Geometry: final body of the model. Coordinates: model frame, mm. Face numbers are marked on the shaded views. A direction names the side the tool comes from. Give positions to 0.01 mm unless a question says otherwise; leave off trailing zeros. Loops run counter-clockwise (first coordinate to the right, second up) from the corner with the lowest first, then second, coordinate; pieces in that order, holes last.
1. Section B-B, the plane z = 10.5. Output: boundary loops of the cut face in (x, y).
2. First-contact query: P1, Ø4, axis at x = -30.5, y = 10.5, coming from the -Z side; P2, Ø2, axis at x = -40.5, y = 1.5, coming from the -Z side; P3, Ø11.5, axis at y = 9.65, z = 15.68, coming from the +X side; P4, Ø2, axis at x = -32.5, y = 16.5, coming from the -Z side. Flat tips, straight axial feed; report the tip coordinate or a pass-through.
3. Material intervals for line 1 along Z through (x, y) = (-38, 0.5); line 2 along Z through (x, y) = (-38, 18.75); line 3 along Y through (x, z) = (-41, 26.5), sorted ascending.
4. Section A-A, the plane y = 11.75. Output: boundary loops of the cut face in (x, z).
5. Draft query along Y for the marked faces 1, 2 and 3. Return one class per face: +Y half, -Y half, draft (parallel to the pull), parting line (faces both ways), or undercut.
6. Access query for the marked faces 4, 5 and 6. Directions: +Z, -Z, +X, -X, +Y, -Y. A direction counts if a zero-diameter tool reaches every point of the face in a straight line with its end or side. Return the directions, or none.
7. Section C-C, the plane y = -2. Output: boundary loops of the cut face in (x, z), then the cut area to 3 significant figures.
8. Section D-D, the plane z = 15.5. Output: boundary loops of the cut face in (x, y), then the cut area to 3 significant figures.
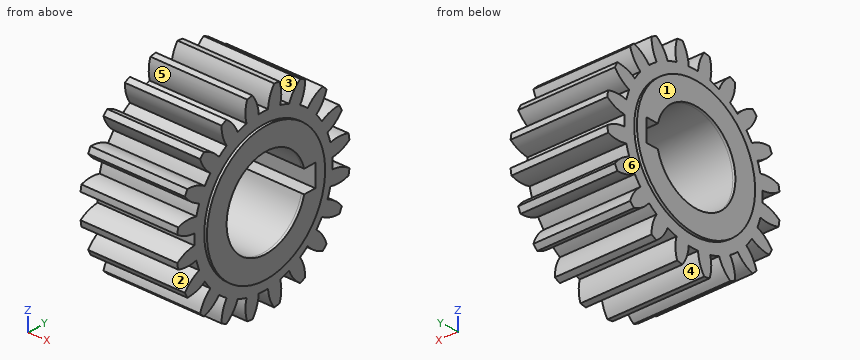
from build123d import *

# Parameters (mm, degrees)
SPUR_START             = -42.145535126
SPUR_GEAR_AI_OUTLINE_R = 6.35
SPUR_GEAR_AI_DEPTH     = 13.97
SKETCH1_W              = 3.175
SKETCH1_H              = 3.175
CUT_EXTRUDE1_DEPTH     = 41.258239372
SKETCH2_R              = 9.525
BOSS_EXTRUDE1_DEPTH    = 0.381
BOSS_EXTRUDE2_START    = 0.381
SKETCH3_R              = 9.525
BOSS_EXTRUDE2_DEPTH    = 0.381


# Read off the part's stored shape, not the designer's step: spur gear_ai
with BuildPart() as part:
    # spur gear_ai outline → spur gear_ai (new body)
    with BuildSketch(Plane.YZ.offset(SPUR_START)):
        with BuildLine():
            ThreePointArc((21.89573329, 8.949900066), (22.10150024, 9.338497576), (22.294935451, 9.733378421))
            ThreePointArc((22.294935451, 9.733378421), (21.269289936, 10.804918767), (19.977842952, 11.534516))
            ThreePointArc((19.977842952, 11.534516), (20.234833052, 12.242868992), (20.443283136, 12.966993591))
            ThreePointArc((20.443283136, 12.966993591), (21.916932187, 12.79815666), (23.376532451, 13.062191702))
            ThreePointArc((23.376532451, 13.062191702), (23.452145215, 13.495355381), (23.514088141, 13.93068415))
            ThreePointArc((23.514088141, 13.93068415), (22.207517114, 14.632837684), (20.7538201, 14.927646821))
            ThreePointArc((20.7538201, 14.927646821), (20.779339097, 15.680744858), (20.7538201, 16.433842895))
            ThreePointArc((20.7538201, 16.433842895), (22.207517114, 16.728652032), (23.514088141, 17.430805566))
            ThreePointArc((23.514088141, 17.430805566), (23.452145215, 17.866134334), (23.376532451, 18.299298013))
            ThreePointArc((23.376532451, 18.299298013), (21.916932187, 18.563333056), (20.443283136, 18.394496125))
            ThreePointArc((20.443283136, 18.394496125), (20.234833052, 19.118620724), (19.977842952, 19.826973715))
            ThreePointArc((19.977842952, 19.826973715), (21.269289936, 20.556570948), (22.294935451, 21.628111294))
            ThreePointArc((22.294935451, 21.628111294), (22.10150024, 22.022992139), (21.89573329, 22.41158965))
            ThreePointArc((21.89573329, 22.41158965), (20.425979632, 22.21166061), (19.07662958, 21.595704547))
            ThreePointArc((19.07662958, 21.595704547), (18.654614962, 22.219973346), (18.191309741, 22.814242767))
            ThreePointArc((18.191309741, 22.814242767), (19.194090867, 23.907210035), (19.83841354, 25.243247358))
            ThreePointArc((19.83841354, 25.243247358), (19.53242083, 25.559026591), (19.216641597, 25.865019301))
            ThreePointArc((19.216641597, 25.865019301), (17.880604274, 25.220696628), (16.787637006, 24.217915502))
            ThreePointArc((16.787637006, 24.217915502), (16.193367585, 24.681220723), (15.569098786, 25.103235341))
            ThreePointArc((15.569098786, 25.103235341), (16.185054849, 26.452585393), (16.384983889, 27.922339051))
            ThreePointArc((16.384983889, 27.922339051), (15.996386378, 28.128106001), (15.601505533, 28.321541212))
            ThreePointArc((15.601505533, 28.321541212), (14.529965187, 27.295895697), (13.800367954, 26.004448713))
            ThreePointArc((13.800367954, 26.004448713), (13.092014963, 26.261438813), (12.367890364, 26.469888897))
            ThreePointArc((12.367890364, 26.469888897), (12.536727295, 27.943537948), (12.272692252, 29.403138212))
            ThreePointArc((12.272692252, 29.403138212), (11.839528573, 29.478750976), (11.404199805, 29.540693902))
            ThreePointArc((11.404199805, 29.540693902), (10.702046271, 28.234122875), (10.407237134, 26.780425861))
            ThreePointArc((10.407237134, 26.780425861), (9.654139097, 26.805944858), (8.90104106, 26.780425861))
            ThreePointArc((8.90104106, 26.780425861), (8.606231923, 28.234122875), (7.904078389, 29.540693902))
            ThreePointArc((7.904078389, 29.540693902), (7.46874962, 29.478750976), (7.035585941, 29.403138212))
            ThreePointArc((7.035585941, 29.403138212), (6.771550899, 27.943537948), (6.94038783, 26.469888897))
            ThreePointArc((6.94038783, 26.469888897), (6.216263231, 26.261438813), (5.507910239, 26.004448713))
            ThreePointArc((5.507910239, 26.004448713), (4.778313006, 27.295895697), (3.70677266, 28.321541212))
            ThreePointArc((3.70677266, 28.321541212), (3.311891815, 28.128106001), (2.923294305, 27.922339051))
            ThreePointArc((2.923294305, 27.922339051), (3.123223344, 26.452585393), (3.739179408, 25.103235341))
            ThreePointArc((3.739179408, 25.103235341), (3.114910608, 24.681220723), (2.520641187, 24.217915502))
            ThreePointArc((2.520641187, 24.217915502), (1.427673919, 25.220696628), (0.091636597, 25.865019301))
            ThreePointArc((0.091636597, 25.865019301), (-0.224142637, 25.559026591), (-0.530135347, 25.243247358))
            ThreePointArc((-0.530135347, 25.243247358), (0.114187326, 23.907210035), (1.116968452, 22.814242767))
            ThreePointArc((1.116968452, 22.814242767), (0.653663231, 22.219973346), (0.231648613, 21.595704547))
            ThreePointArc((0.231648613, 21.595704547), (-1.117701439, 22.21166061), (-2.587455096, 22.41158965))
            ThreePointArc((-2.587455096, 22.41158965), (-2.793222046, 22.022992139), (-2.986657258, 21.628111294))
            ThreePointArc((-2.986657258, 21.628111294), (-1.961011743, 20.556570948), (-0.669564759, 19.826973715))
            ThreePointArc((-0.669564759, 19.826973715), (-0.926554858, 19.118620723), (-1.135004943, 18.394496125))
            ThreePointArc((-1.135004943, 18.394496125), (-2.608653994, 18.563333056), (-4.068254258, 18.299298013))
            ThreePointArc((-4.068254258, 18.299298013), (-4.143867021, 17.866134334), (-4.205809948, 17.430805566))
            ThreePointArc((-4.205809948, 17.430805566), (-2.899238921, 16.728652032), (-1.445541907, 16.433842895))
            ThreePointArc((-1.445541907, 16.433842895), (-1.471060903, 15.680744858), (-1.445541907, 14.927646821))
            ThreePointArc((-1.445541907, 14.927646821), (-2.899238921, 14.632837684), (-4.205809948, 13.93068415))
            ThreePointArc((-4.205809948, 13.93068415), (-4.143867021, 13.495355381), (-4.068254258, 13.062191702))
            ThreePointArc((-4.068254258, 13.062191702), (-2.608653994, 12.79815666), (-1.135004943, 12.966993591))
            ThreePointArc((-1.135004943, 12.966993591), (-0.926554858, 12.242868992), (-0.669564759, 11.534516))
            ThreePointArc((-0.669564759, 11.534516), (-1.961011743, 10.804918767), (-2.986657258, 9.733378421))
            ThreePointArc((-2.986657258, 9.733378421), (-2.793222046, 9.338497576), (-2.587455096, 8.949900066))
            ThreePointArc((-2.587455096, 8.949900066), (-1.117701439, 9.149829105), (0.231648613, 9.765785169))
            ThreePointArc((0.231648613, 9.765785169), (0.653663231, 9.141516369), (1.116968452, 8.547246948))
            ThreePointArc((1.116968452, 8.547246948), (0.114187326, 7.45427968), (-0.530135347, 6.118242358))
            ThreePointArc((-0.530135347, 6.118242358), (-0.224142637, 5.802463124), (0.091636597, 5.496470414))
            ThreePointArc((0.091636597, 5.496470414), (1.427673919, 6.140793087), (2.520641187, 7.143574213))
            ThreePointArc((2.520641187, 7.143574213), (3.114910608, 6.680268992), (3.739179408, 6.258254374))
            ThreePointArc((3.739179408, 6.258254374), (3.123223344, 4.908904322), (2.923294305, 3.439150665))
            ThreePointArc((2.923294305, 3.439150665), (3.311891815, 3.233383715), (3.70677266, 3.039948503))
            ThreePointArc((3.70677266, 3.039948503), (4.778313006, 4.065594018), (5.507910239, 5.357041002))
            ThreePointArc((5.507910239, 5.357041002), (6.216263231, 5.100050903), (6.94038783, 4.891600818))
            ThreePointArc((6.94038783, 4.891600818), (6.771550899, 3.417951767), (7.035585941, 1.958351503))
            ThreePointArc((7.035585941, 1.958351503), (7.46874962, 1.882738739), (7.904078389, 1.820795813))
            ThreePointArc((7.904078389, 1.820795813), (8.606231923, 3.12736684), (8.90104106, 4.581063854))
            ThreePointArc((8.90104106, 4.581063854), (9.654139097, 4.555544858), (10.407237134, 4.581063854))
            ThreePointArc((10.407237134, 4.581063854), (10.702046271, 3.12736684), (11.404199805, 1.820795813))
            ThreePointArc((11.404199805, 1.820795813), (11.839528573, 1.882738739), (12.272692252, 1.958351503))
            ThreePointArc((12.272692252, 1.958351503), (12.536727295, 3.417951767), (12.367890364, 4.891600818))
            ThreePointArc((12.367890364, 4.891600818), (13.092014962, 5.100050903), (13.800367954, 5.357041002))
            ThreePointArc((13.800367954, 5.357041002), (14.529965187, 4.065594018), (15.601505533, 3.039948503))
            ThreePointArc((15.601505533, 3.039948503), (15.996386378, 3.233383715), (16.384983889, 3.439150665))
            ThreePointArc((16.384983889, 3.439150665), (16.185054849, 4.908904322), (15.569098786, 6.258254374))
            ThreePointArc((15.569098786, 6.258254374), (16.193367585, 6.680268992), (16.787637006, 7.143574213))
            ThreePointArc((16.787637006, 7.143574213), (17.880604274, 6.140793087), (19.216641597, 5.496470414))
            ThreePointArc((19.216641597, 5.496470414), (19.53242083, 5.802463124), (19.83841354, 6.118242358))
            ThreePointArc((19.83841354, 6.118242358), (19.194090867, 7.45427968), (18.191309741, 8.547246948))
            ThreePointArc((18.191309741, 8.547246948), (18.654614962, 9.141516369), (19.07662958, 9.765785169))
            ThreePointArc((19.07662958, 9.765785169), (20.425979632, 9.149829105), (21.89573329, 8.949900066))
        make_face()
        with Locations((9.654139097, 15.680744858)):
            Circle(SPUR_GEAR_AI_OUTLINE_R, mode=Mode.SUBTRACT)
    extrude(amount=SPUR_GEAR_AI_DEPTH)

    # Sketch1 → Cut-Extrude1 (cut, through all)
    with BuildSketch(Plane(origin=(-28.175535126, 0, 0), x_dir=(0, 0, -1), z_dir=(1, 0, 0))):
        with Locations((-15.680744858, 16.004139097)):
            Rectangle(SKETCH1_W, SKETCH1_H)
    extrude(amount=-CUT_EXTRUDE1_DEPTH, mode=Mode.SUBTRACT)

    # Sketch2 → Boss-Extrude1 (add)
    with BuildSketch(Plane(origin=(-28.175535126, 0, 0), x_dir=(0, 0, -1), z_dir=(1, 0, 0))):
        with Locations(Location((-15.680744858, 9.654139097, 0), (0, 0, 180))):
            Circle(SKETCH2_R)
        with BuildLine():
            Line((-14.093244858, 17.591639097), (-17.268244858, 17.591639097))
            Line((-17.268244858, 17.591639097), (-17.268244858, 15.802500159))
            ThreePointArc((-17.268244858, 15.802500159), (-15.680744858, 3.304139097), (-14.093244858, 15.802500159))
            Line((-14.093244858, 15.802500159), (-14.093244858, 17.591639097))
        make_face(mode=Mode.SUBTRACT)
    extrude(amount=BOSS_EXTRUDE1_DEPTH)

    # Sketch3 → Boss-Extrude2 (add)
    with BuildSketch(Plane.ZY.offset(42.145535126).offset(BOSS_EXTRUDE2_START)):
        with Locations((15.680744858, 9.654139097)):
            Circle(SKETCH3_R)
        with BuildLine():
            Line((14.093244858, 15.802500159), (14.093244858, 17.591639097))
            Line((14.093244858, 17.591639097), (17.268244858, 17.591639097))
            Line((17.268244858, 17.591639097), (17.268244858, 15.802500159))
            ThreePointArc((17.268244858, 15.802500159), (15.680744858, 3.304139097), (14.093244858, 15.802500159))
        make_face(mode=Mode.SUBTRACT)
    extrude(amount=-BOSS_EXTRUDE2_DEPTH)


solid = part.part
Answers below:
1. outline: (-42.53, 1.66) - (-42.15, 1.66) - (-42.15, -2.32) - (-28.18, -2.32) - (-28.18, 1.66) - (-27.79, 1.66) - (-27.79, 5.98) - (-42.53, 5.98) - close; (-42.53, 13.33) - (-27.79, 13.33) - (-27.79, 17.65) - (-28.18, 17.65) - (-28.18, 21.63) - (-42.15, 21.63) - (-42.15, 17.65) - (-42.53, 17.65) - close
2. P1: stops at z = 1.82
2. P2: stops at z = 5.64
2. P3: passes through
2. P4: stops at z = 3.04
3. line 1: z = 5.64 to 7.95, 9.36 to 22, 23.41 to 25.72
3. line 2: z = 5.67 to 8.02, 9.27 to 22.09, 23.34 to 25.69
3. line 3: y = 3.11 to 5.29, 6.93 to 12.38, 14.02 to 16.2
4. outline: (-42.53, 6.39) - (-42.15, 6.39) - (-42.15, 1.87) - (-28.18, 1.87) - (-28.18, 6.39) - (-27.79, 6.39) - (-27.79, 9.69) - (-42.53, 9.69) - close; (-42.53, 21.67) - (-27.79, 21.67) - (-27.79, 24.97) - (-28.18, 24.97) - (-28.18, 29.49) - (-42.15, 29.49) - (-42.15, 24.97) - (-42.53, 24.97) - close
5. face 1: draft
5. face 2: -Y half
5. face 3: undercut
6. face 4: -Z, +X, -X
6. face 5: +X, -X
6. face 6: -X
7. outline: (-42.15, 8.98) - (-28.18, 8.98) - (-28.18, 10.77) - (-42.15, 10.77) - close; (-42.15, 12.81) - (-28.18, 12.81) - (-28.18, 14.87) - (-42.15, 14.87) - close; (-42.15, 16.49) - (-28.18, 16.49) - (-28.18, 18.55) - (-42.15, 18.55) - close; (-42.15, 20.59) - (-28.18, 20.59) - (-28.18, 22.38) - (-42.15, 22.38) - close
7. area: 108 mm2
8. outline: (-42.53, 0.13) - (-42.15, 0.13) - (-42.15, -1.47) - (-28.18, -1.47) - (-28.18, 0.13) - (-27.79, 0.13) - (-27.79, 3.31) - (-42.53, 3.31) - close; (-42.53, 17.59) - (-27.79, 17.59) - (-27.79, 19.18) - (-28.18, 19.18) - (-28.18, 20.78) - (-42.15, 20.78) - (-42.15, 19.18) - (-42.53, 19.18) - close
8. area: 115 mm2
